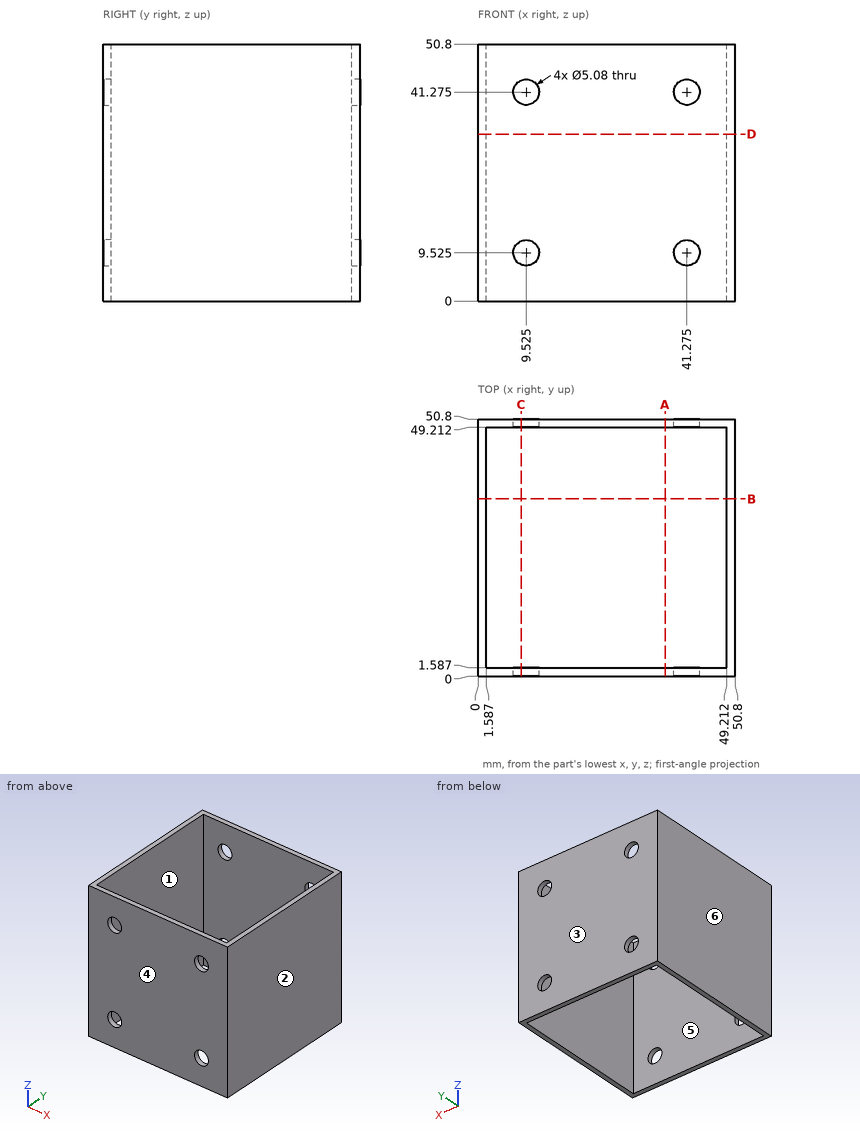
For this review, use the dimensioned drawing (mm, ordinates from the lowest corner) and the shaded views. A direction names the side the tool comes from. Give positions to 0.01 mm unless a question says otherwise; leave off trailing zeros. Write each loop counter-clockwise with the first axis right and the second up, starting at its lowest first coordinate (ties: lowest second). Pieces come first, ordered by that corner, then holes. Notation, with made-up numbers: M 76,53 L 86,53 A22 ccw 86,64 Z; hole C 7.5,-39.5 d7. An arc over 180 degrees is marked long. Answer as a JSON object with one key per item and string values. Group by question number.
Item 1: For probe 1 along X at (y, z) = (11, 44.5), list the stretches that pass through material, from the lowest coordinate up. Write a range as [from, to].
Item 2: For pin 1 Ø4 at (x, z) = (41.275, 41.275) entering from -Y, flat-tipped, find the tip position at first contact; note if it passes through.
Item 3: Consider section D-D on z = 33. Write out the cut boundary in (x, y).
Item 4: Consider section C-C on x = 8.5. Write out the cut boundary in (y, z).
Item 5: Draft analysis for pull direction Y (two halves, no side actions). For the marked faces 3, 4, 5 and 6, state which applies: +Y half, -Y half, draft (parallel to the pull), parting line (faces both ways), or undercut.
Item 6: Consider section A-A on x = 37. Write out the cut boundary in (y, z).
Item 7: Tool access review of the marked faces 1 and 2: name each direction out of +Z, -Z, +X, -X, +Y, -Y from which nothing blocks a thin tool from reaching the whole face with its end or side.
Check result:
{
 "1": {"probe 1": "x = [0, 1.59], [49.21, 50.8]"},
 "2": {"pin 1": "passes through"},
 "3": {"outline": "M 0,0 L 50.8,0 L 50.8,50.8 L 0,50.8 Z; hole M 1.59,1.59 L 49.21,1.59 L 49.21,49.21 L 1.59,49.21 Z"},
 "4": {"outline": "M 0,0 L 1.59,0 L 1.59,7.2 L 0,7.2 Z; M 0,11.85 L 1.59,11.85 L 1.59,38.95 L 0,38.95 Z; M 0,43.6 L 1.59,43.6 L 1.59,50.8 L 0,50.8 Z; M 49.21,0 L 50.8,0 L 50.8,7.2 L 49.21,7.2 Z; M 49.21,11.85 L 50.8,11.85 L 50.8,38.95 L 49.21,38.95 Z; M 49.21,43.6 L 50.8,43.6 L 50.8,50.8 L 49.21,50.8 Z"},
 "5": {"face 3": "+Y half", "face 4": "-Y half", "face 5": "undercut", "face 6": "draft"},
 "6": {"outline": "M 0,0 L 1.59,0 L 1.59,50.8 L 0,50.8 Z; M 49.21,0 L 50.8,0 L 50.8,50.8 L 49.21,50.8 Z"},
 "7": {"face 1": "+Z, -Z", "face 2": "+Z, -Z, +X, +Y, -Y"}
}
